Model file for the job. Use its own axes, mm. Round coordinates to 2 decimals unless told otherwise and drop trailing zeros. Write each loop counter-clockwise with the first axis right and the second up, starting at its lowest first coordinate (ties: lowest second). Pieces come first, ordered by that corner, then holes.
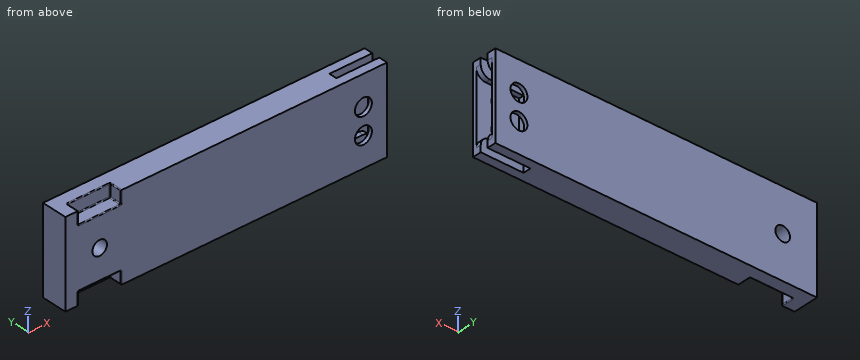
```python
from build123d import *

# Parameters (mm, degrees)
SKETCH1_W            = 20
SKETCH1_H            = 6
BOSS_EXTRUDE1_DEPTH  = 75
M3_CLEARANCE_HOLE1_D = 3.4
SKETCH4_R            = 1.975
CUT_EXTRUDE1_DEPTH   = 76.901251637
CUT_EXTRUDE2_DEPTH   = 10
SKETCH6_W            = 10
SKETCH6_H            = 3
CUT_EXTRUDE3_DEPTH   = 3
FILLET1_R            = 0.2
FILLET2_R            = 2.2


with BuildPart() as part:
    # Sketch1 → Boss-Extrude1 (new body)
    with BuildSketch(Plane(origin=(0, 0, 0), x_dir=(0, 0, -1), z_dir=(1, 0, 0))):
        with Locations((0, -3)):
            Rectangle(SKETCH1_W, SKETCH1_H)
    extrude(amount=BOSS_EXTRUDE1_DEPTH)

    # M3 Clearance Hole1 (through all)
    with Locations(Plane(origin=(0, 0, 0), x_dir=(1, 0, 0), z_dir=(0, 1, 0))):
        with Locations((8, 0)):
            Hole(M3_CLEARANCE_HOLE1_D / 2)

    # Sketch4 → Cut-Extrude1 (cut, through all)
    with BuildSketch(Plane(origin=(0, 0, 0), x_dir=(1, 0, 0), z_dir=(0, 1, 0))):
        with Locations(Location((69.5, 3, 0), (0, 0, 270))):
            Circle(SKETCH4_R)
        with Locations(Location((69.5, -3, 0), (0, 0, 270))):
            Circle(SKETCH4_R)
    extrude(amount=-CUT_EXTRUDE1_DEPTH, mode=Mode.SUBTRACT)

    # Sketch5 → Cut-Extrude2 (cut)
    with BuildSketch(Plane(origin=(75, 0, 0), x_dir=(0, 0, -1), z_dir=(1, 0, 0))):
        Polygon((-10, -3.925), (-6.3, -3.925), (-6.3, -5.125), (6.3, -5.125), (6.3, -3.925), (10, -3.925), (10, -2.075), (6.3, -2.075), (6.3, -0.875), (-6.3, -0.875), (-6.3, -2.075), (-10, -2.075), align=None)
    extrude(amount=-CUT_EXTRUDE2_DEPTH, mode=Mode.SUBTRACT)

    # Sketch6 → Cut-Extrude3 (cut)
    with BuildSketch(Plane.XZ.offset(6)):
        with Locations((8, 8.5)):
            Rectangle(SKETCH6_W, SKETCH6_H)
        with Locations((8, -8.5)):
            Rectangle(SKETCH6_W, SKETCH6_H)
    extrude(amount=-CUT_EXTRUDE3_DEPTH, mode=Mode.SUBTRACT)

    # Fillet1
    fillet1_edges = [part.edges().sort_by_distance(p)[0] for p in [
        (3, -3, 8.5),
        (3, -4.5, 7),
        (8, -3, 10),
        (3, -4.5, 10),
        (13, -3, 8.5),
        (13, -4.5, 10),
        (8, -3, 7),
        (13, -4.5, 7),
        (3, -6, 8.5),
        (8, -6, 7),
        (13, -6, 8.5),
        (13, -3, -8.5),
        (13, -4.5, -7),
        (8, -3, -10),
        (13, -4.5, -10),
        (3, -3, -8.5),
        (3, -4.5, -10),
        (8, -3, -7),
        (3, -4.5, -7),
        (13, -6, -8.5),
        (8, -6, -7),
        (3, -6, -8.5),
    ]]
    fillet(fillet1_edges, radius=FILLET1_R)

    # Fillet2
    fillet2_edges = [part.edges().sort_by_distance(p)[0] for p in [
        (75, -1.475, -6.3),
        (75, -1.475, 6.3),
        (75, -4.525, 6.3),
        (75, -4.525, -6.3),
    ]]
    fillet(fillet2_edges, radius=FILLET2_R)


solid = part.part
```
1) Cut at D-D on x = 69.5. Give the number of separate pieces and of enclosed holes in the cut face, and give its area (3 significant figures).
2) Flat gauge pins, fed straight in: pin 1 Ø0.8 at (x, z) = (9.5, -8.5) entering from -Y; pin 2 Ø0.8 at (y, z) = (-4.5, 8) entering from -X. Where does each tip first touch, or does it go through?
3) Cut at B-B on z = 3. List the corners of the cut face in (x, y) (3 decimals), and give its area (3 significant figures).
4) Wall check: probe 1 along X at (y, z) = (-0.6, -3) (3 decimals); probe 2 along X at (y, z) = (-5.1, 8.75); probe 3 along X at (y, z) = (-4.8, 6.25). Give the ranges that are in metal, low to high.
5) Cut at C-C on z = 0. List the corners of the cut face in (x, y) (3 decimals), and give its area (3 significant figures).
6) Cut at A-A on x = 8. List the corners of the cut face in (y, z), and give its area (3 significant figures).
Result sheet:
1. separate pieces: 6
1. enclosed holes: 0
1. area: 38.9 mm2
2. pin 1: stops at y = -3
2. pin 2: stops at x = 0
3. outline: (0, -6) - (67.525, -6) - (67.525, -5.125) - (65, -5.125) - (65, -0.875) - (67.525, -0.875) - (67.525, 0) - (0, 0) - close; (71.475, -6) - (75, -6) - (75, -5.125) - (71.475, -5.125) - close; (71.475, -0.875) - (75, -0.875) - (75, 0) - (71.475, 0) - close
3. area: 401 mm2
4. probe 1: x = 0 to 67.525, 71.475 to 75
4. probe 2: x = 0 to 3, 13 to 75
4. probe 3: x = 0 to 65
5. outline: (0, -6) - (6.3, -6) - (6.3, 0) - (0, 0) - close; (9.7, -6) - (75, -6) - (75, -5.125) - (65, -5.125) - (65, -0.875) - (75, -0.875) - (75, 0) - (9.7, 0) - close
5. area: 387 mm2
6. outline: (-6, -6.8) arc R0.2 ccw to (-5.8, -7) - (-3.2, -7) arc R0.2 cw to (-3, -7.2) - (-3, -9.8) arc R0.2 ccw to (-2.8, -10) - (0, -10) - (0, -1.7) - (-6, -1.7) - close; (-6, 1.7) - (0, 1.7) - (0, 10) - (-2.8, 10) arc R0.2 ccw to (-3, 9.8) - (-3, 7.2) arc R0.2 cw to (-3.2, 7) - (-5.8, 7) arc R0.2 ccw to (-6, 6.8) - close
6. area: 81.6 mm2
